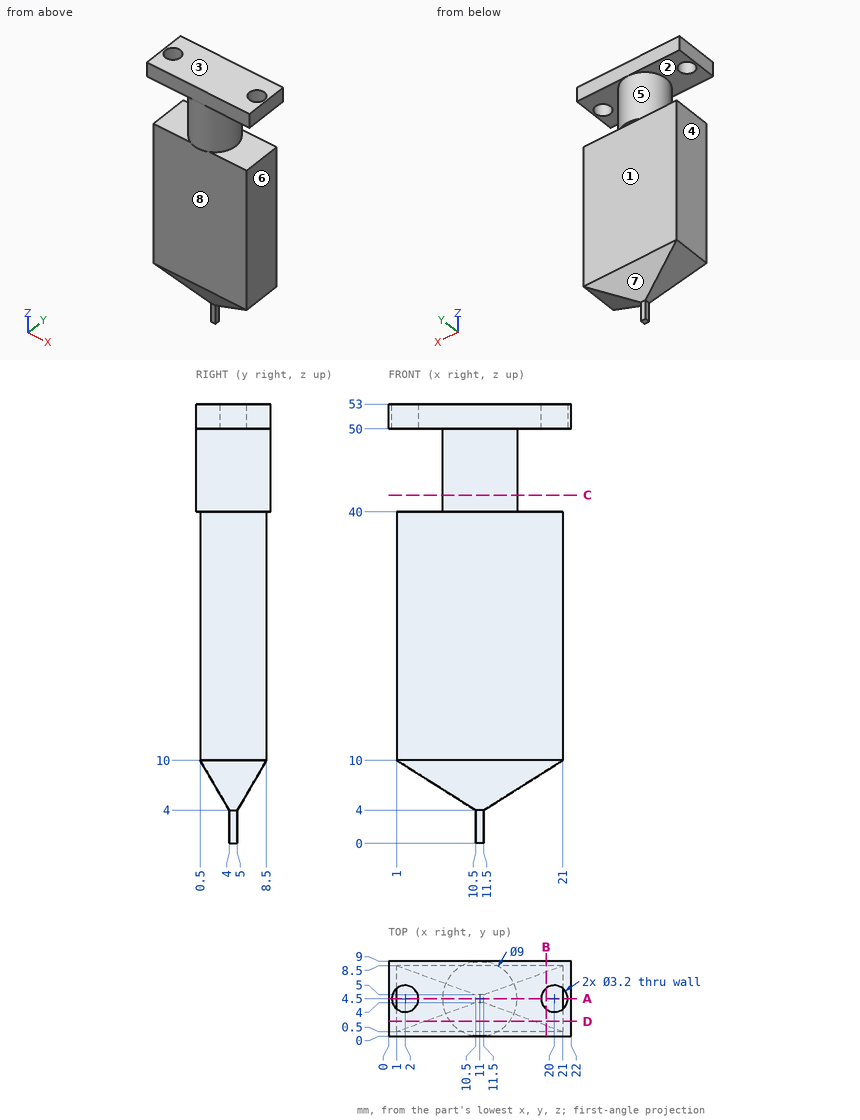
Geometry check sheet. Reference: drawing and pictorial views, mm from the part's lowest x, y, z. A direction names the side the tool comes from. Round coordinates to 2 decimals unless told otherwise and drop trailing zeros. Write each loop counter-clockwise with the first axis right and the second up, starting at its lowest first coordinate (ties: lowest second). Pieces come first, ordered by that corner, then holes.
(1) Access from +Z, -Z, +X, -X, +Y, -Y to the whole of each face (thin tool, end or side, straight path). Record for the marked faces 4, 5, 6, 7 and 8.
Returned:
face 4: -Z, -X, +Y, -Y
face 5: none
face 6: -Z, +X, +Y, -Y
face 7: -Z, +X, -X, +Y
face 8: -Z, +X, -X, -Y
(2) Section check B-B (x = 19). Enter the section's corners in (y, z).
Returned:
outline: (0, 50) - (3.25, 50) - (3.25, 53) - (0, 53) - close; (0.5, 10) - (1.24, 8.74) - (7.76, 8.74) - (8.5, 10) - (8.5, 40) - (0.5, 40) - close; (5.75, 50) - (9, 50) - (9, 53) - (5.75, 53) - close
(3) Material ranges on line 1 (Y direction, x = 20, z = 51.05); line 2 (Y direction, x = 20.25, z = 12); line 3 (Z direction, x = 21, y = 8.75), recorded low to high.
Returned:
line 1: y = 0 to 2.9, 6.1 to 9
line 2: y = 0.5 to 8.5
line 3: z = 50 to 53
(4) Section check C-C (z = 42). Enter the section's corners in (x, y).
Returned:
outline: circle Ø9 at (11, 4.5)
(5) Section check D-D (y = 1.75). Enter the section's corners in (x, z), plus the area to 3 significant figures.
Returned:
outline: (0, 50) - (7.44, 50) - (7.44, 40) - (1, 40) - (1, 10) - (4.39, 7.86) - (17.61, 7.86) - (21, 10) - (21, 40) - (14.56, 40) - (14.56, 50) - (22, 50) - (22, 53) - (0, 53) - close
area: 773 mm2
(6) Depth check by flat-ended pin: pin 1 Ø1 at (x, y) = (16.5, 2) entering from -Z; pin 2 Ø3 at (x, y) = (3.5, 5) entering from -Z; pin 3 Ø12 at (x, z) = (11, 13) entering from +Y. Enter the tip coordinate at first touch or a pass-through.
Returned:
pin 1: stops at z = 6.91
pin 2: stops at z = 7.47
pin 3: stops at y = 8.5
(7) Mould release check, pull along Z, two halves, no side actions. Record for the marked faces 1, 2 and 3: pulls with the +Z half, pulls with the -Z half, needs draft (parallel to the pull), parting line crosses it, or undercut.
Returned:
face 1: needs draft
face 2: undercut
face 3: pulls with the +Z half
(8) Section check A-A (y = 4.5). Enter the section's corners in (x, z).
Returned:
outline: (0, 50) - (0.4, 50) - (0.4, 53) - (0, 53) - close; (1, 10) - (10.5, 4) - (10.5, 0) - (11.5, 0) - (11.5, 4) - (21, 10) - (21, 40) - (15.5, 40) - (15.5, 50) - (18.4, 50) - (18.4, 53) - (3.6, 53) - (3.6, 50) - (6.5, 50) - (6.5, 40) - (1, 40) - close; (21.6, 50) - (22, 50) - (22, 53) - (21.6, 53) - close
